```python
from build123d import *

# Parameters (mm, degrees)
SKETCH005_W     = 111
SKETCH005_H     = 41
PAD002_DEPTH    = 3.6
SKETCH006_R     = 5
SKETCH006_R_2   = 1.6
PAD003_DEPTH    = 2
SKETCH007_R     = 1
POCKET001_DEPTH = 5
SKETCH008_W     = 5
SKETCH008_H     = 41
SKETCH008_R     = 1.6
PAD004_DEPTH    = 1


with BuildPart() as part:
    # Sketch005 → Pad002 (new body)
    with BuildSketch(Plane.XY):
        with BuildLine():
            Line((0, -3), (111, -3))
            ThreePointArc((111, -3), (113.12132, -2.12132), (114, 0))
            Line((114, 0), (114, 41))
            ThreePointArc((114, 41), (113.12132, 43.12132), (111, 44))
            Line((111, 44), (0, 44))
            ThreePointArc((0, 44), (-2.12132, 43.12132), (-3, 41))
            Line((-3, 41), (-3, 0))
            ThreePointArc((-3, 0), (-2.12132, -2.12132), (0, -3))
        make_face()
        with Locations((55.5, 20.5)):
            Rectangle(SKETCH005_W, SKETCH005_H, mode=Mode.SUBTRACT)
    extrude(amount=PAD002_DEPTH)

    # Sketch006 → Pad003 (join)
    with BuildSketch(Plane.XY):
        with Locations((4.7, 25.9)):
            Circle(SKETCH006_R)
        with Locations((4.7, 25.9)):
            Circle(SKETCH006_R_2, mode=Mode.SUBTRACT)
        with Locations((106.3, 25.9)):
            Circle(SKETCH006_R)
        with Locations((106.3, 25.9)):
            Circle(SKETCH006_R_2, mode=Mode.SUBTRACT)
        with Locations((52.96, 25.9)):
            Circle(SKETCH006_R)
        with Locations((52.96, 25.9)):
            Circle(SKETCH006_R_2, mode=Mode.SUBTRACT)
    extrude(amount=PAD003_DEPTH)

    # Sketch007 → Pocket001 (cut)
    with BuildSketch(Plane.XY.offset(2)):
        with Locations((0, 41)):
            Circle(SKETCH007_R)
        with Locations((111, 41)):
            Circle(SKETCH007_R)
        with Locations((111, 0)):
            Circle(SKETCH007_R)
        Circle(SKETCH007_R)
    extrude(amount=POCKET001_DEPTH, mode=Mode.SUBTRACT)

    # Sketch008 → Pad004 (join)
    with BuildSketch(Plane.XY):
        with Locations((52.96, 20.5)):
            Rectangle(SKETCH008_W, SKETCH008_H)
        with Locations((52.96, 25.9)):
            Circle(SKETCH008_R, mode=Mode.SUBTRACT)
    extrude(amount=PAD004_DEPTH)


solid = part.part
```
Input: part model. Units: mm. Frame: model coordinates. A direction names the side the tool comes from. Give positions to 0.01 mm unless a question says otherwise; leave off trailing zeros. Order: outer loops, then holes, each group sorted by start corner. A loop starts at its lowest first (then second) coordinate and runs counter-clockwise, first axis right, second up. Notation, with made-up numbers: (85, 60.5) - (112, 60.5) arc R24 cw to (112, 99.5) - close; hole circle Ø11 at (81.5, 16). An arc over 180 degrees is marked (long way). Put each result on its own line as item: value.
Item 1: Ray query, L1, parallel to X at y = 8, z = 0.7; L2, parallel to Y at x = 52.96, z = 1.5; L3, parallel to Y at x = 83, z = 1.95. Return the intervals inside material, ascending. Write a range as from..to.
Found:
L1: x = -3..0, 50.46..55.46, 111..114
L2: y = -3..0, 20.9..24.3, 27.5..30.9, 41..44
L3: y = -3..0, 41..44
Item 2: Section query D-D, the plane x = 52.96. Return loops of the section in (y, z).
Found:
outline: (-3, 0) - (24.3, 0) - (24.3, 2) - (20.9, 2) - (20.9, 1) - (0, 1) - (0, 3.6) - (-3, 3.6) - close; (27.5, 0) - (44, 0) - (44, 3.6) - (41, 3.6) - (41, 1) - (30.9, 1) - (30.9, 2) - (27.5, 2) - close
Item 3: Section query A-A, the plane x = 74.5. Return loops of the section in (y, z), then the cut area to 3 significant figures.
Found:
outline: (-3, 0) - (0, 0) - (0, 3.6) - (-3, 3.6) - close; (41, 0) - (44, 0) - (44, 3.6) - (41, 3.6) - close
area: 21.6 mm^2
Item 4: Contact query for flat-ended pins moving along their axis: pin 1 (5 mm diameter, centred on x = 3.5, y = 25, fed in from +Z); pin 2 (3.5 mm diameter, centred on x = 4.7, y = 25.9, fed in from -Z); pin 3 (1 mm diameter, centred on x = 50, y = 8.5, fed in from +Z). Output: stop coordinate, or through.
Found:
pin 1: stops at z = 2
pin 2: stops at z = 0
pin 3: stops at z = 1
Item 5: Access query for faces 4 (the flat face through (114, 20, 2)), 5 (the cylindrical face through (111.73, 41.683, 2.789)). Directions: +Z, -Z, +X, -X, +Y, -Y. A direction counts if a zero-diameter tool reaches every point of the face in a straight line with its end or side. Return the directions, or none.
Found:
face 4: +Z, -Z, +X, +Y, -Y
face 5: +Z
Item 6: Draft query along X for faces 1 (the cylindrical face through (113.1, -2.14, 1.77)), 2 (the cylindrical face through (-0.73, -0.683, 2.789)), 3 (the flat face through (56, 44, 2)). Return one class per face: +X half, -X half, draft (parallel to the pull), parting line (faces both ways), or undercut.
Found:
face 1: +X half
face 2: undercut
face 3: draft
Item 7: Section query C-C, the plane x = 4.7. Return loops of the section in (y, z), then the cut area to 3 significant figures.
Found:
outline: (-3, 0) - (0, 0) - (0, 3.6) - (-3, 3.6) - close; (20.9, 0) - (24.3, 0) - (24.3, 2) - (20.9, 2) - close; (27.5, 0) - (30.9, 0) - (30.9, 2) - (27.5, 2) - close; (41, 0) - (44, 0) - (44, 3.6) - (41, 3.6) - close
area: 35.2 mm^2
Item 8: Section query B-B, the plane y = 11.5. Return loops of the section in (x, z), then the cut area to 3 significant figures.
Found:
outline: (-3, 0) - (0, 0) - (0, 3.6) - (-3, 3.6) - close; (50.46, 0) - (55.46, 0) - (55.46, 1) - (50.46, 1) - close; (111, 0) - (114, 0) - (114, 3.6) - (111, 3.6) - close
area: 26.6 mm^2
